Check sheet for the modelled part. Datum: model origin and axes. Units: mm. A direction names the side the tool comes from. Round coordinates to 2 decimals unless told otherwise and drop trailing zeros. Write each loop counter-clockwise with the first axis right and the second up, starting at its lowest first coordinate (ties: lowest second). Pieces come first, ordered by that corner, then holes. Notation, with made-up numbers: M 48.25,68 L 101.25,68 A27 ccw 101.25,87 Z; hole C -11,36.5 d9. An arc over 180 degrees is marked long. One line per item, written item: value.
from build123d import *

# Parameters (mm, degrees)
F1_DEPTH = 18
F3_DEPTH = 6


with BuildPart() as f1:
    # F0 (on Top) → F1 (new body)
    with BuildSketch(Plane.XY):
        Polygon((834.8224465267, -191.4757991363), (-270.6217704598, 374.7018082726), (-321.7972505834, -102.5623431511), (630.5432843246, -590.3245270833), align=None)
    extrude(amount=F1_DEPTH)

    # F2 (on face) → F3 (cut)
    with BuildSketch(Plane(origin=(0, 0, 0), x_dir=(1, 0, 0), z_dir=(0, 0, -1))):
        Polygon((-271.9921794431, -361.9213306116), (829.3521314793, 202.1564195902), (826.6169739555, 207.4967298172), (-272.6773839347, -355.5310917811), align=None)
    extrude(amount=-F3_DEPTH, mode=Mode.SUBTRACT)


solid = f1.part
Q1. Sectioned sample at A-A on y = 312.5. Enter the section's corners in (x, z).
Completed:
outline: M -277.29,0 L -188.66,0 L -188.66,6 L -175.5,6 L -175.5,0 L -149.17,0 L -149.17,18 L -277.29,18 Z
Q2. Sectioned sample at C-C on z = 15.25. Enter the section's corners in (x, y), and give its area (3 significant figures).
Completed:
outline: M -321.8,-102.56 L 630.54,-590.32 L 834.82,-191.48 L -270.62,374.7 Z
area: 518,000 mm^2
Q3. Access from +Z, -Z, +X, -X, +Y, -Y to the whole of each face (thin tool, end or side, straight path). Record for faces 4 (the flat face through (248, -101, 18)), 5 (the flat face through (153, 139, 6)).
Completed:
face 4: +Z, +X, -X, +Y, -Y
face 5: -Z
Q4. Draft check along Y on faces 1 (the flat face through (289.84, 87.65, 8.87)), 2 (the flat face through (279, 88, 0)), 3 (the flat face through (284.66, 70.08, 2.96)). Enter one of: pulls with the +Y half, pulls with the -Y half, needs draft (parallel to the pull), parting line crosses it, or undercut.
Completed:
face 1: pulls with the +Y half
face 2: needs draft
face 3: undercut
Q5. Sectioned sample at B-B on x = 706. Enter the section's corners in (y, z).
Completed:
outline: M -443,0 L -145.72,0 L -145.72,6 L -138.98,6 L -138.98,0 L -125.5,0 L -125.5,18 L -443,18 Z
Q6. Scan lines: line 1 (Y direction, x = 784, z = 5.5); line 2 (Y direction, x = 658.5, z = 3.5); line 3 (X direction, y = -166.5, z = 2.5). Record each from-to range of solid material in increasing order. Write a range as [from, to].
Completed:
line 1: [-290.71, -185.67], [-178.93, -165.45]
line 2: [-535.74, -121.39], [-114.65, -101.17]
line 3: [-196.96, 746.57], [759.73, 786.06]
Q7. Sectioned sample at D-D on y = -309. Enter the section's corners in (x, z).
Completed:
outline: M 81.27,0 L 774.63,0 L 774.63,18 L 81.27,18 Z
Q8. Depth check by flat-ended pin: P1, Ø4, axis at y = -126, z = 14, coming from the +X side; P2, Ø6, axis at x = 352, z = 14.5, coming from the -Y side; P3, Ø6, axis at x = -196.5, z = 4.5, coming from the -Y side. Enter the tip coordinate at first touch or a pass-through.
Completed:
P1: x = 710.89
P2: y = -449.2
P3: y = -168.27
